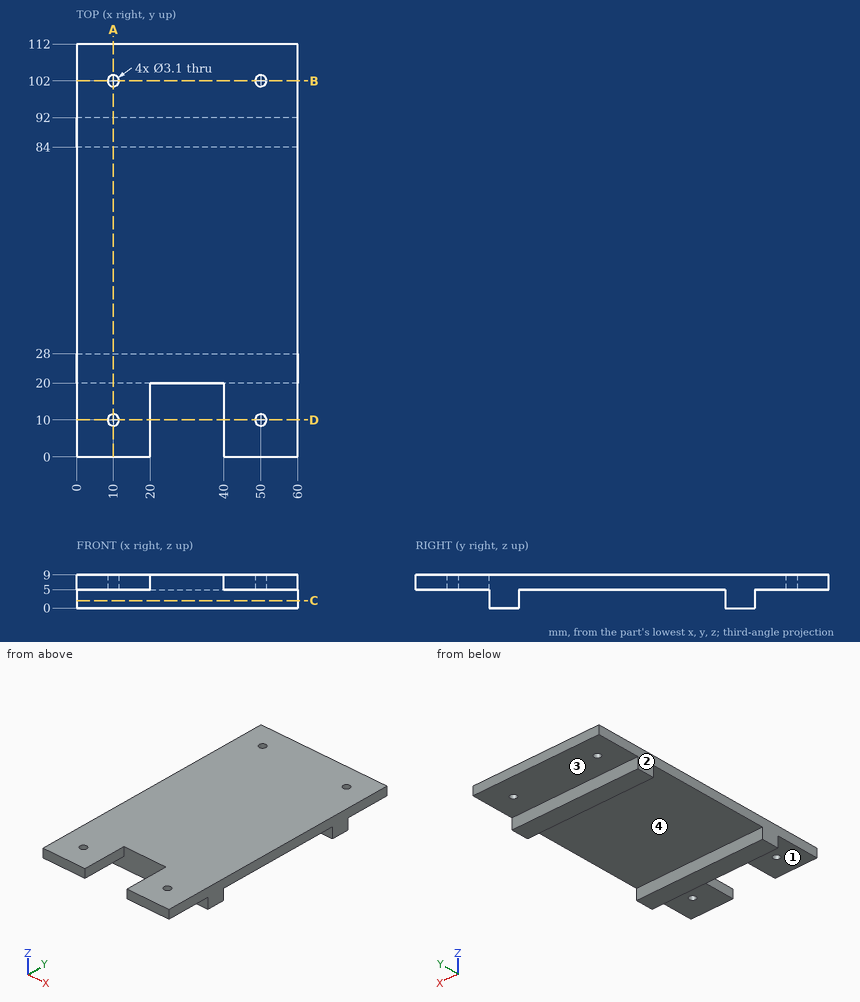
Input: dimensioned drawing with shaded views. Units: mm. Origin: part minimum x, y, z. A direction names the side the tool comes from. Round coordinates to 2 decimals unless told otherwise and drop trailing zeros. Loops run counter-clockwise (first coordinate to the right, second up) from the corner with the lowest first, then second, coordinate; pieces in that order, holes last. Notation, with made-up numbers: M 57,7 L 100,7 A33 cw 100,42 Z; hole C 75.25,24.5 d10. An arc over 180 degrees is marked long. Return JSON: item names as keys, results as strings. Group by question number.
1. Mould query, pull axis Y, two halves, no side actions, for the marked faces 3 and 4. Classes: released by +Y, released by -Y, zero draft, split by the parting line, or undercut.
2. Pin query (flat end, axial travel): pin 1 (2 mm diameter, centred on x = 41.5, y = 15.5, fed in from -Z); pin 2 (1.5 mm diameter, centred on x = 26.5, z = 3, fed in from +Y); pin 3 (4.5 mm diameter, centred on x = 37, z = 3, fed in from -Y). Return the tip coordinate at first contact, or that it passes through.
3. Material intervals for line 1 along X through (y, z) = (102, 6.75); line 2 along Y through (x, z) = (10, 6.45); line 3 along Y through (x, z) = (25, 4), sorted ascending. Write a range as from..to.
4. Section query A-A on x = 10. Output: boundary loops of the cut face in (y, z), and give its area (3 significant figures).
5. Section query B-B on y = 102. Output: boundary loops of the cut face in (x, z).
6. Section query C-C on z = 2. Output: boundary loops of the cut face in (x, y), and give its area (3 significant figures).
7. Section query D-D on y = 10. Output: boundary loops of the cut face in (x, z), and give its area (3 significant figures).
8. Reachability of the marked faces 1 and 2 from +Z, -Z, +X, -X, +Y, -Y: full face, straight path, thin tool, end or side. Return the list, or none.
Checks:
{
 "1": {"face 3": "zero draft", "face 4": "undercut"},
 "2": {"pin 1": "stops at z = 5", "pin 2": "stops at y = 92", "pin 3": "stops at y = 20"},
 "3": {"line 1": "x = 0..8.45, 11.55..48.45, 51.55..60", "line 2": "y = 0..8.45, 11.55..100.45, 103.55..112", "line 3": "y = 20..28, 84..92"},
 "4": {"outline": "M 0,5 L 8.45,5 L 8.45,9 L 0,9 Z; M 11.55,5 L 20,5 L 20,0 L 28,0 L 28,5 L 84,5 L 84,0 L 92,0 L 92,5 L 100.45,5 L 100.45,9 L 11.55,9 Z; M 103.55,5 L 112,5 L 112,9 L 103.55,9 Z", "area": "503 mm²"},
 "5": {"outline": "M 0,5 L 8.45,5 L 8.45,9 L 0,9 Z; M 11.55,5 L 48.45,5 L 48.45,9 L 11.55,9 Z; M 51.55,5 L 60,5 L 60,9 L 51.55,9 Z"},
 "6": {"outline": "M 0,20 L 60,20 L 60,28 L 0,28 Z; M 0,84 L 60,84 L 60,92 L 0,92 Z", "area": "960 mm²"},
 "7": {"outline": "M 0,5 L 8.45,5 L 8.45,9 L 0,9 Z; M 11.55,5 L 20,5 L 20,9 L 11.55,9 Z; M 40,5 L 48.45,5 L 48.45,9 L 40,9 Z; M 51.55,5 L 60,5 L 60,9 L 51.55,9 Z", "area": "135 mm²"},
 "8": {"face 1": "-Z, +X, -X, -Y", "face 2": "+Z, -Z, -X, +Y, -Y"}
}
